Geometry: final body of the model. Coordinates: model frame, mm. Round coordinates to 2 decimals unless told otherwise and drop trailing zeros. Write each loop counter-clockwise with the first axis right and the second up, starting at its lowest first coordinate (ties: lowest second). Pieces come first, ordered by that corner, then holes. Notation, with made-up numbers: M 23.25,29 L 70.25,29 A23 cw 70.25,50 Z; hole C 4,14.25 d10. An arc over 180 degrees is marked long. Use one line per item in the form item = value. Start each with the question number.
Item 1: Section query A-A (z = 102). Return loops of the section in (x, y), and give its area (3 significant figures).
Item 2: Section query B-B (y = -125). Return loops of the section in (x, z), and give its area (3 significant figures).
Item 3: Pin query (flat end, axial travel): pin 1 Ø2 at (x, y) = (1.5, -12) entering from +Z; pin 2 Ø2 at (x, y) = (2.5, -165) entering from -Z; pin 3 Ø2 at (x, z) = (2, -2.5) entering from +Y. Return the tip coordinate at first contact, or that it passes through.
Item 4: Ray query, probe 1 along Y at (x, z) = (0.85, 8.5); probe 2 along Z at (x, y) = (3, -104); probe 3 along Z at (x, y) = (2.25, -113). Return the intervals inside material, ascending.
Item 5: Section query C-C (z = 170.5). Return loops of the section in (x, y), and give its area (3 significant figures).
from build123d import *

# Parameters (mm, degrees)
F1_DEPTH = 4
F2_R     = 60
F3_DEPTH = 25


with BuildPart() as f1:
    # F0 (on Right) → F1 (new body)
    with BuildSketch(Plane.YZ):
        with BuildLine():
            Line((-20, 0), (0, 0))
            Line((0, 0), (0, 40))
            Line((0, 40), (-4, 40))
            Line((-4, 40), (-4, 85))
            Line((-4, 85), (0, 85))
            Line((0, 85), (0, 175))
            Line((0, 175), (-4, 175))
            Line((-4, 175), (-4, 220))
            Line((-4, 220), (0, 220))
            Line((0, 220), (0, 250))
            Line((0, 250), (-21.25, 250))
            Line((-21.25, 250), (-21.25, 254))
            Line((-21.25, 254), (-63.75, 254))
            Line((-63.75, 254), (-63.75, 250))
            Line((-63.75, 250), (-79.5, 250))
            Line((-79.5, 250), (-79.5, 254))
            Line((-79.5, 254), (-98.672283, 240.056522))
            ThreePointArc((-98.672283, 240.056522), (-99.775105, 233.071983), (-106.759644, 234.174805))
            Line((-106.759644, 234.174805), (-254, 127.090909))
            Line((-254, 127.090909), (-250, 127.090909))
            Line((-250, 127.090909), (-250, 85))
            Line((-250, 85), (-254, 85))
            Line((-254, 85), (-254, 40))
            Line((-254, 40), (-250, 40))
            Line((-250, 40), (-250, 0))
            Line((-250, 0), (-230, 0))
            Line((-230, 0), (-230, -4))
            Line((-230, -4), (-190, -4))
            Line((-190, -4), (-190, 0))
            Line((-190, 0), (-150, 0))
            Line((-150, 0), (-150, -4))
            Line((-150, -4), (-100, -4))
            Line((-100, -4), (-100, 0))
            Line((-100, 0), (-60, 0))
            Line((-60, 0), (-60, -4))
            Line((-60, -4), (-20, -4))
            Line((-20, -4), (-20, 0))
        make_face()
    extrude(amount=F1_DEPTH)

    # F2 (on face) → F3 (cut)
    with BuildSketch(Plane(origin=(0, 0, 0), x_dir=(0, -1, 0), z_dir=(-1, 0, 0))):
        with Locations((125, 97.391762)):
            Circle(F2_R)
    extrude(amount=-F3_DEPTH, mode=Mode.SUBTRACT)


solid = f1.part
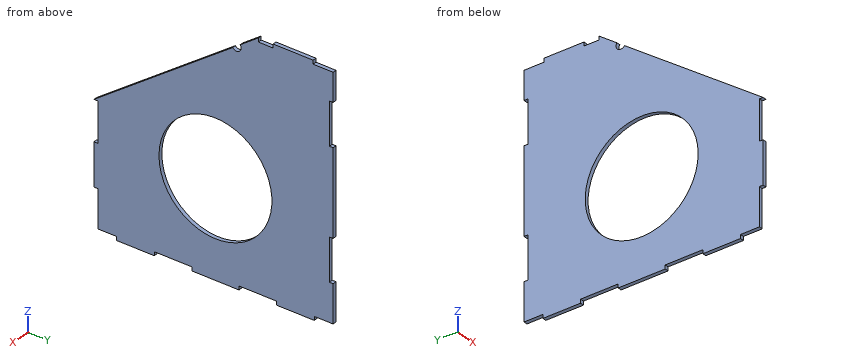
Working result:
q1.outline = M 0,-250 L 4,-250 L 4,-184.82 L 0,-184.82 Z; M 0,-65.18 L 4,-65.18 L 4,0 L 0,0 Z
q1.area = 521 mm²
q2.outline = M 0,-4 L 4,-4 L 4,37.39 L 0,37.39 Z; M 0,157.39 L 4,157.39 L 4,220.91 L 0,220.91 Z
q2.area = 420 mm²
q3.pin_1 = 250
q3.pin_2 = 0
q3.pin_3 = -20
q4.probe_1 = -250 to 0
q4.probe_2 = -4 to 41.19, 153.6 to 232.28
q4.probe_3 = -4 to 38.6, 156.18 to 229.64
q5.outline = M 0,-194.31 L 4,-194.31 L 4,0 L 0,0 Z
q5.area = 777 mm²
